The figure shows three views and two pictorial views of one solid part (mm, origin at its lowest corner). Answer the questions. Coordinates: 2 decimals unless noted, no trailing zeros. Write each loop counter-clockwise with the first axis right and the second up, starting at its lowest first coordinate (ties: lowest second). Pieces come first, ordered by that corner, then holes.
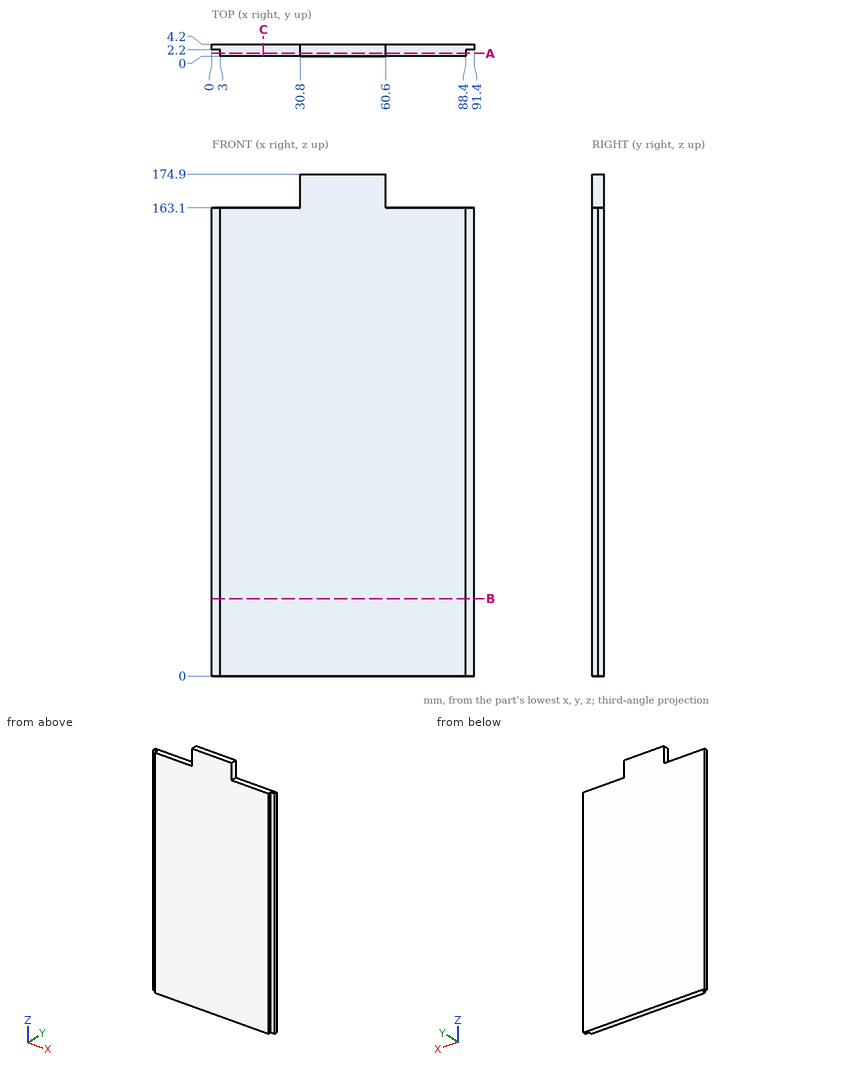
Q1. Given pin 1 (2 mm diameter, centred on x = 10, y = 1.5, fed in from +Z); pin 2 (0.9 mm diameter, centred on x = 1, z = 118, fed in from -Y); pin 3 (1.8 mm diameter, centred on y = 1, z = 105.5, fed in from -X), each flat-ended and moving along its own axis, determine where each tip first touches the part or whether it passes through.
Answers below:
pin 1: stops at z = 163.1
pin 2: stops at y = 2.2
pin 3: stops at x = 3
Q2. The part is cut by section A-A, the plane y = 0.9. Write down the section's boundary in (x, z), then the cut area to 3 significant figures.
Answers below:
outline: (3, 0) - (88.4, 0) - (88.4, 163.1) - (60.6, 163.1) - (60.6, 174.9) - (30.8, 174.9) - (30.8, 163.1) - (3, 163.1) - close
area: 14,300 mm2
Q3. Find the intervals of material crossed by probe 1 along Z at (x, y) = (66, 1.1); probe 2 along X at (y, z) = (1.5, 114), in increasing order.
Answers below:
probe 1: z = 0 to 163.1
probe 2: x = 3 to 88.4
Q4. The part is cut by section C-C, the plane x = 18. Write down the section's boundary in (y, z), then the cut area to 3 significant figures.
Answers below:
outline: (0, 0) - (4.2, 0) - (4.2, 163.1) - (0, 163.1) - close
area: 685 mm2
Q5. The part is cut by section B-B, the plane z = 27. Write down the section's boundary in (x, y).
Answers below:
outline: (0, 2.2) - (3, 2.2) - (3, 0) - (88.4, 0) - (88.4, 2.2) - (91.4, 2.2) - (91.4, 4.2) - (0, 4.2) - close
